Geometry check sheet. Reference: drawing and pictorial views, mm from the part's lowest x, y, z. Give positions to 0.01 mm unless a question says otherwise; leave off trailing zeros. Write each loop counter-clockwise with the first axis right and the second up, starting at its lowest first coordinate (ties: lowest second). Pieces come first, ordered by that corner, then holes.
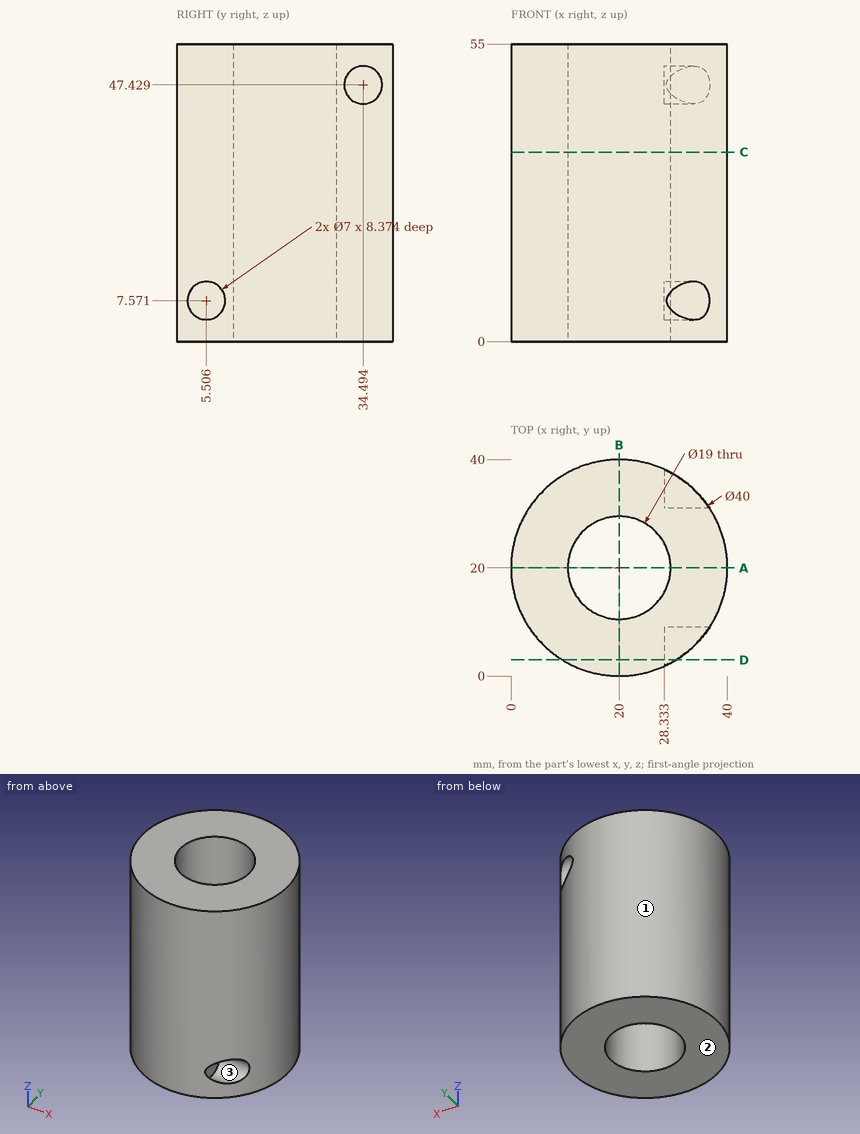
Item 1: Depth check by flat-ended pin: pin 1 (5.5 mm diameter, centred on y = 34.49, z = 47.43, fed in from +X); pin 2 (12 mm diameter, centred on y = 32.5, z = 34.5, fed in from +X) (1 decimal); pin 3 (4 mm diameter, centred on y = 12, z = 42, fed in from -X). Enter the tip coordinate at first touch or a pass-through.
Answer key:
pin 1: stops at x = 28.33
pin 2: stops at x = 38.9
pin 3: stops at x = 0.92
Item 2: Scan lines: line 1 along Y through (x, z) = (20, 7.5); line 2 along X through (y, z) = (17.5, 13) (1 decimal); line 3 along Z through (x, y) = (34.5, 8) (1 decimal). Record each from-to range of solid material in increasing order.
Answer key:
line 1: y = 0 to 10.5, 29.5 to 40
line 2: x = 0.2 to 10.8, 29.2 to 39.8
line 3: z = 0 to 5.1, 10 to 55
Item 3: Sectioned sample at D-D on y = 3. Record the cut outline in (x, z) (1 decimal), then the cut area to 3 significant figures.
Answer key:
outline: (9.5, 0) - (30.5, 0) - (30.5, 5.1) - (28.3, 5.1) - (28.3, 10) - (30.5, 10) - (30.5, 55) - (9.5, 55) - close
area: 1,150 mm2
Item 4: Sectioned sample at C-C on z = 35. Record the cut outline in (x, y), then the cut area to 3 significant figures.
Answer key:
outline: circle Ø40 at (20, 20); hole circle Ø19 at (20, 20)
area: 973 mm2
Item 5: Release check for a two-part mould opening along Y. For the marked faces 1, 2 and 3 record: released by +Y, released by -Y, zero draft, split by the parting line, or undercut.
Answer key:
face 1: split by the parting line
face 2: zero draft
face 3: undercut
Item 6: Sectioned sample at A-A on y = 20. Record the cut outline in (x, z), then the cut area to 4 significant figures.
Answer key:
outline: (0, 0) - (10.5, 0) - (10.5, 55) - (0, 55) - close; (29.5, 0) - (40, 0) - (40, 55) - (29.5, 55) - close
area: 1,155 mm2
